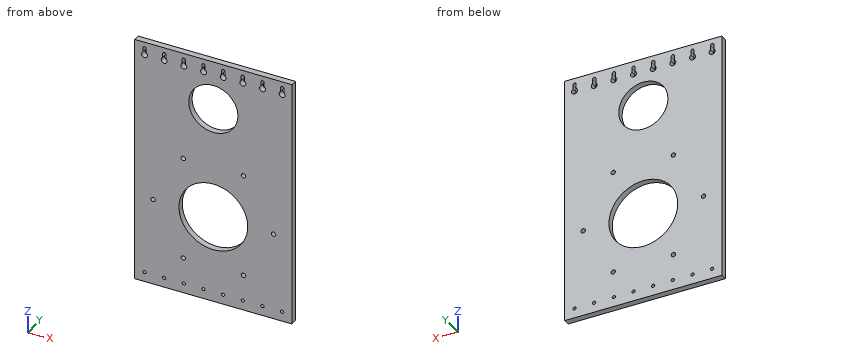
from build123d import *

# Parameters (mm, degrees)
SKETCH1_W           = 160
SKETCH1_H           = 255
SKETCH1_R           = 35
SKETCH1_R_2         = 25
SKETCH1_R_3         = 2.25
SKETCH1_R_4         = 1.65
BOSS_EXTRUDE1_DEPTH = 6.35
CUT_EXTRUDE1_REACH  = 303.107
SKETCH2_R           = 3


with BuildPart() as part:
    # Sketch1 → Boss-Extrude1 (new body)
    with BuildSketch(Plane(origin=(0, 0, 0), x_dir=(1, 0, 0), z_dir=(0, 1, 0))):
        with Locations((80, 127.5)):
            Rectangle(SKETCH1_W, SKETCH1_H)
        with Locations(Location((80, 165, 0), (0, 0, 270))):
            Circle(SKETCH1_R, mode=Mode.SUBTRACT)
        with Locations(Location((80, 50, 0), (0, 0, 270))):
            Circle(SKETCH1_R_2, mode=Mode.SUBTRACT)
        with Locations(Location((141.25, 165, 0), (0, 0, 270))):
            Circle(SKETCH1_R_3, mode=Mode.SUBTRACT)
        with Locations(Location((110.625, 111.955944018, 0), (0, 0, 270))):
            Circle(SKETCH1_R_3, mode=Mode.SUBTRACT)
        with Locations(Location((49.375, 111.955944018, 0), (0, 0, 270))):
            Circle(SKETCH1_R_3, mode=Mode.SUBTRACT)
        with Locations(Location((18.75, 165, 0), (0, 0, 270))):
            Circle(SKETCH1_R_3, mode=Mode.SUBTRACT)
        with Locations(Location((49.375, 218.044055982, 0), (0, 0, 270))):
            Circle(SKETCH1_R_3, mode=Mode.SUBTRACT)
        with Locations(Location((110.625, 218.044055982, 0), (0, 0, 270))):
            Circle(SKETCH1_R_3, mode=Mode.SUBTRACT)
        with Locations(Location((10, 245, 0), (0, 0, 270))):
            Circle(SKETCH1_R_4, mode=Mode.SUBTRACT)
        with Locations(Location((30, 245, 0), (0, 0, 270))):
            Circle(SKETCH1_R_4, mode=Mode.SUBTRACT)
        with Locations(Location((50, 245, 0), (0, 0, 270))):
            Circle(SKETCH1_R_4, mode=Mode.SUBTRACT)
        with Locations(Location((70, 245, 0), (0, 0, 270))):
            Circle(SKETCH1_R_4, mode=Mode.SUBTRACT)
        with Locations(Location((90, 245, 0), (0, 0, 270))):
            Circle(SKETCH1_R_4, mode=Mode.SUBTRACT)
        with Locations(Location((110, 245, 0), (0, 0, 270))):
            Circle(SKETCH1_R_4, mode=Mode.SUBTRACT)
        with Locations(Location((130, 245, 0), (0, 0, 270))):
            Circle(SKETCH1_R_4, mode=Mode.SUBTRACT)
        with Locations(Location((150, 245, 0), (0, 0, 270))):
            Circle(SKETCH1_R_4, mode=Mode.SUBTRACT)
        with BuildLine():
            Line((8.35, 6.5), (8.35, 13.5))
            ThreePointArc((8.35, 13.5), (10, 15.15), (11.65, 13.5))
            Line((11.65, 13.5), (11.65, 6.5))
            ThreePointArc((11.65, 6.5), (10, 4.85), (8.35, 6.5))
        make_face(mode=Mode.SUBTRACT)
        with BuildLine():
            Line((31.65, 6.5), (31.65, 13.5))
            ThreePointArc((31.65, 13.5), (30, 15.15), (28.35, 13.5))
            Line((28.35, 13.5), (28.35, 6.5))
            ThreePointArc((28.35, 6.5), (30, 4.85), (31.65, 6.5))
        make_face(mode=Mode.SUBTRACT)
        with BuildLine():
            Line((51.65, 6.5), (51.65, 13.5))
            ThreePointArc((51.65, 13.5), (50, 15.15), (48.35, 13.5))
            Line((48.35, 13.5), (48.35, 6.5))
            ThreePointArc((48.35, 6.5), (50, 4.85), (51.65, 6.5))
        make_face(mode=Mode.SUBTRACT)
        with BuildLine():
            Line((71.65, 6.5), (71.65, 13.5))
            ThreePointArc((71.65, 13.5), (70, 15.15), (68.35, 13.5))
            Line((68.35, 13.5), (68.35, 6.5))
            ThreePointArc((68.35, 6.5), (70, 4.85), (71.65, 6.5))
        make_face(mode=Mode.SUBTRACT)
        with BuildLine():
            Line((91.65, 6.5), (91.65, 13.5))
            ThreePointArc((91.65, 13.5), (90, 15.15), (88.35, 13.5))
            Line((88.35, 13.5), (88.35, 6.5))
            ThreePointArc((88.35, 6.5), (90, 4.85), (91.65, 6.5))
        make_face(mode=Mode.SUBTRACT)
        with BuildLine():
            Line((111.65, 6.5), (111.65, 13.5))
            ThreePointArc((111.65, 13.5), (110, 15.15), (108.35, 13.5))
            Line((108.35, 13.5), (108.35, 6.5))
            ThreePointArc((108.35, 6.5), (110, 4.85), (111.65, 6.5))
        make_face(mode=Mode.SUBTRACT)
        with BuildLine():
            Line((131.65, 6.5), (131.65, 13.5))
            ThreePointArc((131.65, 13.5), (130, 15.15), (128.35, 13.5))
            Line((128.35, 13.5), (128.35, 6.5))
            ThreePointArc((128.35, 6.5), (130, 4.85), (131.65, 6.5))
        make_face(mode=Mode.SUBTRACT)
        with BuildLine():
            Line((151.65, 6.5), (151.65, 13.5))
            ThreePointArc((151.65, 13.5), (150, 15.15), (148.35, 13.5))
            Line((148.35, 13.5), (148.35, 6.5))
            ThreePointArc((148.35, 6.5), (150, 4.85), (151.65, 6.5))
        make_face(mode=Mode.SUBTRACT)
    extrude(amount=BOSS_EXTRUDE1_DEPTH)

    # Sketch2 → Cut-Extrude1 (cut, up to next)
    with BuildSketch(Plane(origin=(0, 6.35, 0), x_dir=(1, 0, 0), z_dir=(0, 1, 0)), mode=Mode.PRIVATE) as cut_extrude1_sk1:
        with Locations((150, 13.5)):
            Circle(SKETCH2_R)
    cut_extrude1_tool1 = extrude(cut_extrude1_sk1.sketch, amount=-CUT_EXTRUDE1_REACH, mode=Mode.PRIVATE) & part.part
    # Sketch2 → Cut-Extrude1 (cut, up to next)
    with BuildSketch(Plane(origin=(0, 6.35, 0), x_dir=(1, 0, 0), z_dir=(0, 1, 0)), mode=Mode.PRIVATE) as cut_extrude1_sk2:
        with Locations((130, 13.5)):
            Circle(SKETCH2_R)
    cut_extrude1_tool2 = extrude(cut_extrude1_sk2.sketch, amount=-CUT_EXTRUDE1_REACH, mode=Mode.PRIVATE) & part.part
    # Sketch2 → Cut-Extrude1 (cut, up to next)
    with BuildSketch(Plane(origin=(0, 6.35, 0), x_dir=(1, 0, 0), z_dir=(0, 1, 0)), mode=Mode.PRIVATE) as cut_extrude1_sk3:
        with Locations((110, 13.5)):
            Circle(SKETCH2_R)
    cut_extrude1_tool3 = extrude(cut_extrude1_sk3.sketch, amount=-CUT_EXTRUDE1_REACH, mode=Mode.PRIVATE) & part.part
    # Sketch2 → Cut-Extrude1 (cut, up to next)
    with BuildSketch(Plane(origin=(0, 6.35, 0), x_dir=(1, 0, 0), z_dir=(0, 1, 0)), mode=Mode.PRIVATE) as cut_extrude1_sk4:
        with Locations((90, 13.5)):
            Circle(SKETCH2_R)
    cut_extrude1_tool4 = extrude(cut_extrude1_sk4.sketch, amount=-CUT_EXTRUDE1_REACH, mode=Mode.PRIVATE) & part.part
    # Sketch2 → Cut-Extrude1 (cut, up to next)
    with BuildSketch(Plane(origin=(0, 6.35, 0), x_dir=(1, 0, 0), z_dir=(0, 1, 0)), mode=Mode.PRIVATE) as cut_extrude1_sk5:
        with Locations((70, 13.5)):
            Circle(SKETCH2_R)
    cut_extrude1_tool5 = extrude(cut_extrude1_sk5.sketch, amount=-CUT_EXTRUDE1_REACH, mode=Mode.PRIVATE) & part.part
    # Sketch2 → Cut-Extrude1 (cut, up to next)
    with BuildSketch(Plane(origin=(0, 6.35, 0), x_dir=(1, 0, 0), z_dir=(0, 1, 0)), mode=Mode.PRIVATE) as cut_extrude1_sk6:
        with Locations((50, 13.5)):
            Circle(SKETCH2_R)
    cut_extrude1_tool6 = extrude(cut_extrude1_sk6.sketch, amount=-CUT_EXTRUDE1_REACH, mode=Mode.PRIVATE) & part.part
    # Sketch2 → Cut-Extrude1 (cut, up to next)
    with BuildSketch(Plane(origin=(0, 6.35, 0), x_dir=(1, 0, 0), z_dir=(0, 1, 0)), mode=Mode.PRIVATE) as cut_extrude1_sk7:
        with Locations((30, 13.5)):
            Circle(SKETCH2_R)
    cut_extrude1_tool7 = extrude(cut_extrude1_sk7.sketch, amount=-CUT_EXTRUDE1_REACH, mode=Mode.PRIVATE) & part.part
    # Sketch2 → Cut-Extrude1 (cut, up to next)
    with BuildSketch(Plane(origin=(0, 6.35, 0), x_dir=(1, 0, 0), z_dir=(0, 1, 0)), mode=Mode.PRIVATE) as cut_extrude1_sk8:
        with Locations((10, 13.5)):
            Circle(SKETCH2_R)
    cut_extrude1_tool8 = extrude(cut_extrude1_sk8.sketch, amount=-CUT_EXTRUDE1_REACH, mode=Mode.PRIVATE) & part.part
    add(cut_extrude1_tool1.solids().sort_by_distance((150, 6.35, -13.5))[0], mode=Mode.SUBTRACT)
    add(cut_extrude1_tool2.solids().sort_by_distance((130, 6.35, -13.5))[0], mode=Mode.SUBTRACT)
    add(cut_extrude1_tool3.solids().sort_by_distance((110, 6.35, -13.5))[0], mode=Mode.SUBTRACT)
    add(cut_extrude1_tool4.solids().sort_by_distance((90, 6.35, -13.5))[0], mode=Mode.SUBTRACT)
    add(cut_extrude1_tool5.solids().sort_by_distance((70, 6.35, -13.5))[0], mode=Mode.SUBTRACT)
    add(cut_extrude1_tool6.solids().sort_by_distance((50, 6.35, -13.5))[0], mode=Mode.SUBTRACT)
    add(cut_extrude1_tool7.solids().sort_by_distance((30, 6.35, -13.5))[0], mode=Mode.SUBTRACT)
    add(cut_extrude1_tool8.solids().sort_by_distance((10, 6.35, -13.5))[0], mode=Mode.SUBTRACT)


solid = part.part
Geometry: final body of the model. Coordinates: model frame, mm. Give positions to 0.01 mm unless a question says otherwise; leave off trailing zeros. Write each loop counter-clockwise with the first axis right and the second up, starting at its lowest first coordinate (ties: lowest second). Pieces come first, ordered by that corner, then holes. Notation, with made-up numbers: M -35.5,-25 L 6.5,-25 A16 ccw 6.5,1 Z; hole C 74.5,17.25 d7. An arc over 180 degrees is marked long. Answer in a Markdown table with one row per item. Add a question column.
(1) Section A-A on z = -28. Return loops of the section in (x, y).
(2) Ray query, line 1 (Z direction, x = 130, y = 2.25); line 2 (X direction, y = 4.5, z = -165); line 3 (Z direction, x = 103, y = 4.25). Return the intervals inside material, ascending.
(3) First-contact query: pin 1 (5 mm diameter, centred on x = 130, z = -13.5, fed in from -Y); pin 2 (7 mm diameter, centred on x = 70, z = -13.5, fed in from +Y). Flat tips, straight axial feed; report the tip coordinate or a pass-through.
(4) Section B-B on y = 2. State how many separate pieces and enclosed holes the cut face has, and give its area (3 significant figures).
Result set:
| question | item | result |
|---|---|---|
| 1 | outline | M 0,0 L 68.13,0 L 68.13,6.35 L 0,6.35 Z; M 91.87,0 L 160,0 L 160,6.35 L 91.87,6.35 Z |
| 2 | line 1 | z = -255 to -246.65, -243.35 to -16.5, -4.85 to 0 |
| 2 | line 2 | x = 0 to 16.5, 21 to 45, 115 to 139, 143.5 to 160 |
| 2 | line 3 | z = -255 to -191.38, -138.62 to -59.8, -40.2 to 0 |
| 3 | pin 1 | passes through |
| 3 | pin 2 | stops at y = 6.35 |
| 4 | separate pieces | 1 |
| 4 | enclosed holes | 24 |
| 4 | area | 34,500 mm^2 |
